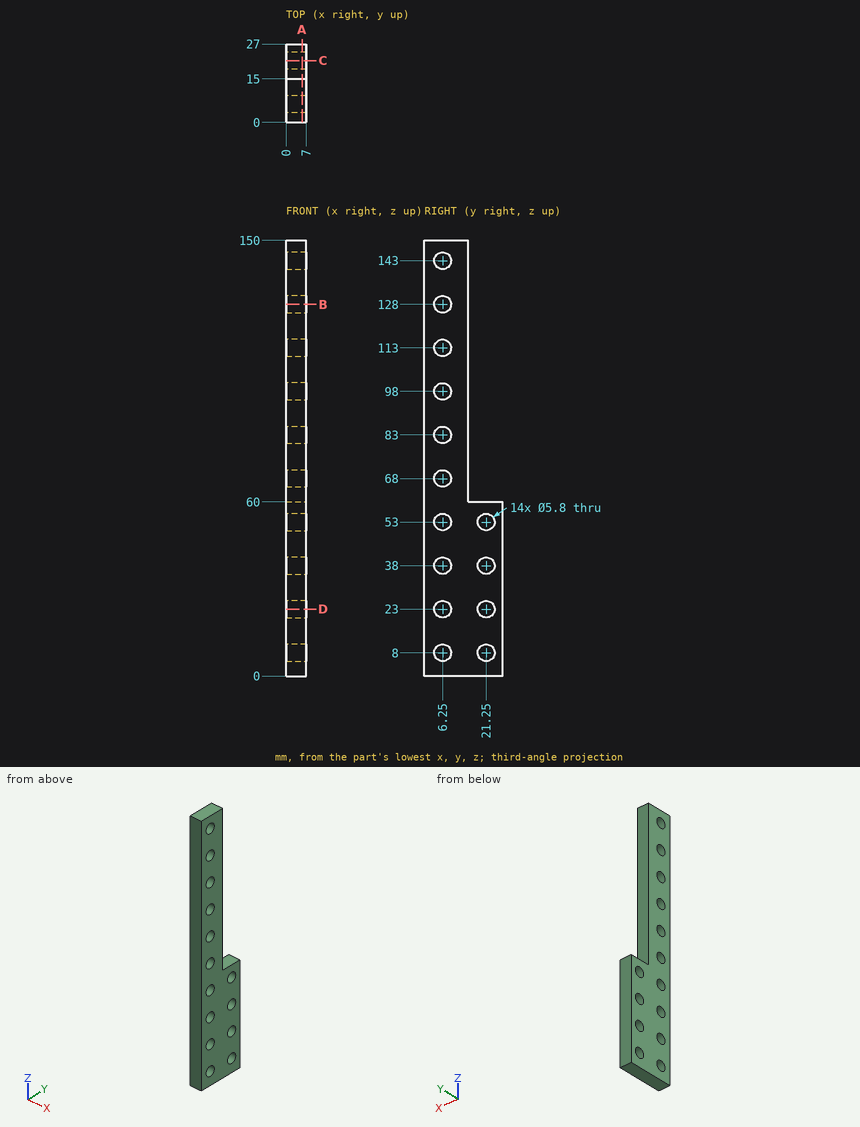
Study the drawing (mm; zero at the part's minimum x, y, z) and answer. Round coordinates to 2 decimals unless told otherwise and drop trailing zeros. Order: outer loops, then holes, each group sorted by start corner. A loop starts at its lowest first (then second) coordinate and runs counter-clockwise, first axis right, second up. Notation, with made-up numbers: (69, 50) -> (126, 50) arc R17 ccw to (126, 74) -> close; hole circle Ø3 at (-35.5, 1.25). An arc over 180 degrees is marked (long way). Answer as CSV lines item,"result". Start each with the question number.
(1) The part is cut by section A-A (x = 5.5). Count the separate pieces of the cut face and the enclosed holes in it, then the cut area to 3 significant figures.
(2) Find the intervals of material crossed by probe 1 along Z at (x, y) = (4.25, 21.25); probe 2 along Y at (x, z) = (2.5, 8); probe 3 along Y at (x, z) = (5, 113), in increasing order. Write a range as from..to.
(3) The part is cut by section D-D (z = 23). Determine the outline of the cut face in (x, y).
(4) The part is cut by section C-C (y = 21.25). Determine the outline of the cut face in (x, z).
(5) The part is cut by section B-B (z = 128). Determine the outline of the cut face in (x, y).
(6) Flat-ended cylindrical pins translate along their axes: pin 1 Ø5 at (y, z) = (6.25, 83) entering from +X; pin 2 Ø1 at (x, z) = (1, 25.5) entering from -Y; pin 3 Ø3.5 at (x, y) = (5, 22.5) entering from +Z; pin 4 Ø2 at (x, z) = (3, 88.5) entering from +Y. Find the tip coordinate at first contact, or state that the pin passes through.
Evaluation:
1,separate pieces,"1"
1,enclosed holes,"14"
1,area,"2,600 mm²"
2,probe 1,"0..5.1, 10.9..20.1, 25.9..35.1, 40.9..50.1, 55.9..60"
2,probe 2,"0..3.35, 9.15..18.35, 24.15..27"
2,probe 3,"0..3.35, 9.15..15"
3,outline,"(0, 0) -> (7, 0) -> (7, 3.35) -> (0, 3.35) -> close; (0, 9.15) -> (7, 9.15) -> (7, 18.35) -> (0, 18.35) -> close; (0, 24.15) -> (7, 24.15) -> (7, 27) -> (0, 27) -> close"
4,outline,"(0, 0) -> (7, 0) -> (7, 5.1) -> (0, 5.1) -> close; (0, 10.9) -> (7, 10.9) -> (7, 20.1) -> (0, 20.1) -> close; (0, 25.9) -> (7, 25.9) -> (7, 35.1) -> (0, 35.1) -> close; (0, 40.9) -> (7, 40.9) -> (7, 50.1) -> (0, 50.1) -> close; (0, 55.9) -> (7, 55.9) -> (7, 60) -> (0, 60) -> close"
5,outline,"(0, 0) -> (7, 0) -> (7, 3.35) -> (0, 3.35) -> close; (0, 9.15) -> (7, 9.15) -> (7, 15) -> (0, 15) -> close"
6,pin 1,"through"
6,pin 2,"y = 0"
6,pin 3,"z = 60"
6,pin 4,"y = 15"
